from build123d import *

# Parameters (mm, degrees)
SKETCH1_W                   = 75
SKETCH1_H                   = 30
BOSS_EXTRUDE1_DEPTH         = 5
SKETCH2_W                   = 25
SKETCH2_H                   = 20
BOSS_EXTRUDE3_DEPTH         = 25.4
SKETCH3_R                   = 3.4925
CUT_EXTRUDE1_DEPTH          = 61.408277578
F_1_4_0_25_DIAMETER_HOLE2_D = 6.35
FILLET2_R                   = 10


with BuildPart() as part:
    # Sketch1 → Boss-Extrude1 (new body)
    with BuildSketch(Plane(origin=(0, 0, 0), x_dir=(1, 0, 0), z_dir=(0, 1, 0))):
        Rectangle(SKETCH1_W, SKETCH1_H)
    extrude(amount=BOSS_EXTRUDE1_DEPTH)

    # Sketch2 → Boss-Extrude3 (add)
    with BuildSketch(Plane(origin=(0, 5, 0), x_dir=(1, 0, 0), z_dir=(0, 1, 0))):
        Rectangle(SKETCH2_W, SKETCH2_H)
    extrude(amount=BOSS_EXTRUDE3_DEPTH)

    # Sketch3 → Cut-Extrude1 (cut, through all)
    with BuildSketch(Plane(origin=(12.5, 0, 0), x_dir=(0, 0, -1), z_dir=(1, 0, 0))):
        with Locations((0, 20.875)):
            Circle(SKETCH3_R)
    extrude(amount=-CUT_EXTRUDE1_DEPTH, mode=Mode.SUBTRACT)

    # 1/4 (0.25) Diameter Hole2 (through all)
    with Locations(Plane(origin=(0, 5, 0), x_dir=(1, 0, 0), z_dir=(0, 1, 0))):
        with Locations((-25, 0), (25, 0)):
            Hole(F_1_4_0_25_DIAMETER_HOLE2_D / 2)

    # Fillet2
    # the kernel refuses this fillet: 10 mm, written as the material it adds along each edge
    with BuildSketch(Plane(origin=(-12.5, 5, 10), x_dir=(0, 0, 1), z_dir=(1, 0, 0)), Plane(origin=(12.5, 5, -10), x_dir=(0, 0, -1), z_dir=(-1, 0, 0))) as fillet2_piece_1:
        with BuildLine():
            CenterArc((10, -8.660254038), FILLET2_R, 120, 60)
            Line((0, -8.660254038), (0, 0))
            Line((0, 0), (5, 0))
        make_face()
    extrude(amount=25)
    # the kernel refuses this fillet: 10 mm, written as the material it takes off along each edge
    with BuildSketch(Plane(origin=(-37.5, -25, -15), x_dir=(1, 0, 0), z_dir=(0, 1, 0)), Plane(origin=(37.5, -25, 15), x_dir=(-1, 0, 0), z_dir=(0, 1, 0))) as fillet2_2_piece_1:
        with BuildLine():
            CenterArc((FILLET2_R, -FILLET2_R), FILLET2_R, 90, 90)
            Line((0, -FILLET2_R), (0, 0))
            Line((0, 0), (FILLET2_R, 0))
        make_face()
    extrude(amount=55, mode=Mode.SUBTRACT)
    with BuildSketch(Plane(origin=(-37.5, -25, 15), x_dir=(1, 0, 0), z_dir=(0, 1, 0)), Plane(origin=(37.5, -25, -15), x_dir=(-1, 0, 0), z_dir=(0, 1, 0))) as fillet2_2_piece_2:
        with BuildLine():
            CenterArc((FILLET2_R, FILLET2_R), FILLET2_R, 180, 90)
            Line((0, FILLET2_R), (0, 0))
            Line((0, 0), (FILLET2_R, 0))
        make_face()
    extrude(amount=55, mode=Mode.SUBTRACT)
    with BuildSketch(Plane(origin=(-37.5, 30.4, 10), x_dir=(0, 0, -1), z_dir=(1, 0, 0)), Plane(origin=(37.5, 30.4, -10), x_dir=(0, 0, 1), z_dir=(-1, 0, 0))) as fillet2_2_piece_3:
        with BuildLine():
            CenterArc((FILLET2_R, -FILLET2_R), FILLET2_R, 90, 90)
            Line((0, -FILLET2_R), (0, 0))
            Line((0, 0), (FILLET2_R, 0))
        make_face()
    extrude(amount=75, mode=Mode.SUBTRACT)


solid = part.part
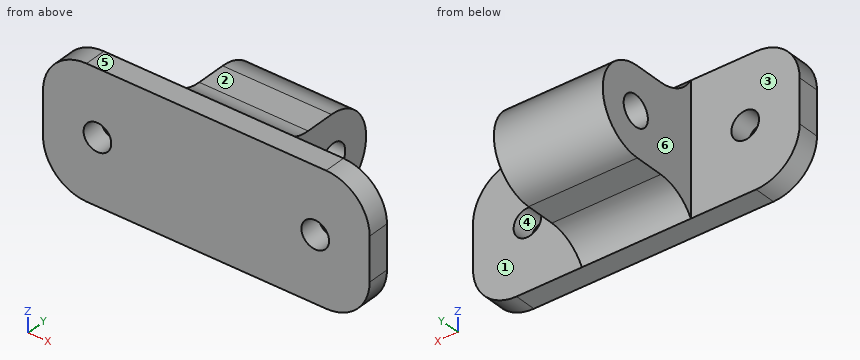
Geometry check sheet. Reference: the model listing, model coordinates, mm. Face numbers are marked on the shaded views. A direction names the side the tool comes from. Give positions to 0.01 mm unless a question says otherwise; leave off trailing zeros. Order: outer loops, then holes, each group sorted by start corner. A loop starts at its lowest first (then second) coordinate and runs counter-clockwise, first axis right, second up.
1. Sectioned sample at C-C (x = -2). Record the boundary of the cut face in (y, z) (1 decimal), then the cut area to 3 significant figures.
Completed:
outline: (0, -15) - (5, -15) arc R10 cw to (13.7, -10) - (20.4, -10) arc R10 ccw to (20.4, 10) - (13.7, 10) arc R10 cw to (5, 15) - (0, 15) - close; hole circle Ø7 at (20.9, 0)
area: 602 mm2
2. Sectioned sample at B-B (z = 0). Record the boundary of the cut face in (x, y) (1 decimal).
Completed:
outline: (-37.5, 0) - (-28.2, 0) - (-28.2, 5) - (-37.5, 5) - close; (-21.8, 0) - (21.8, 0) - (21.8, 5) - (12.5, 5) - (12.5, 17.4) - (-12.5, 17.4) - (-12.5, 5) - (-21.8, 5) - close; (-12.5, 24.4) - (12.5, 24.4) - (12.5, 30.4) - (-12.5, 30.4) - close; (28.2, 0) - (37.5, 0) - (37.5, 5) - (28.2, 5) - close
3. Sectioned sample at A-A (x = -25). Record the boundary of the cut face in (y, z) (3 decimals).
Completed:
outline: (0, -15) - (5, -15) - (5, -3.175) - (0, -3.175) - close; (0, 3.175) - (5, 3.175) - (5, 15) - (0, 15) - close
4. Sectioned sample at D-D (y = 16.5). Record the boundary of the cut face in (x, z).
Completed:
outline: (-12.5, -10) - (12.5, -10) - (12.5, 10) - (-12.5, 10) - close
5. Depth check by flat-ended pin: pin 1 (12.5 mm diameter, centred on x = 25.5, z = 1.5, fed in from +Y); pin 2 (5 mm diameter, centred on y = 26, z = 5.5, fed in from -X); pin 3 (8 mm diameter, centred on y = 20.875, z = 0, fed in from +X). Enter the tip coordinate at first touch or a pass-through.
Completed:
pin 1: stops at y = 5
pin 2: stops at x = -12.5
pin 3: stops at x = 12.5
6. Draft check along X on the marked faces 4, 5 and 6. Enter one of: pulls with the +X half, pulls with the -X half, needs draft (parallel to the pull), parting line crosses it, or undercut.
Completed:
face 4: undercut
face 5: needs draft
face 6: pulls with the -X half
7. Access from +Z, -Z, +X, -X, +Y, -Y to the whole of each face (thin tool, end or side, straight path). Record for the marked faces 1, 2 and 3.
Completed:
face 1: +Z, -Z, +X, +Y
face 2: +Z, +X, -X, +Y
face 3: +Z, -Z, -X, +Y
8. Scan lines: line 1 (Z direction, x = -25, y = 3.2) (3 decimals); line 2 (Y direction, x = -4.5, z = 0); line 3 (Y direction, x = 15, z = 0). Record each from-to range of solid material in increasing order.
Completed:
line 1: z = -15 to -3.175, 3.175 to 15
line 2: y = 0 to 17.38, 24.37 to 30.4
line 3: y = 0 to 5
